Check sheet for the modelled part. Datum: model origin and axes. Units: mm. Face numbers are marked on the shaded views. A direction names the side the tool comes from. Coordinates: 2 decimals unless noted, no trailing zeros. Order: outer loops, then holes, each group sorted by start corner. A loop starts at its lowest first (then second) coordinate and runs counter-clockwise, first axis right, second up.
Autodesk Inventor part; units mm, degrees
ref_plane "YZ Plane" through (0, 0, 0) normal (1, 0, 0) x (0, 1, 0)
ref_plane "XZ Plane" through (0, 0, 0) normal (0, 1, 0) x (-1, 0, 0)
ref_plane "XY Plane" through (0, 0, 0) normal (0, 0, 1) x (1, 0, 0)
sketch "Sketch1" plane through (0, 0, 0) normal (0, 0, 1) x (1, 0, 0)
  line L0 (6.8523, -0.0001) -> (16.3773, -0.0001)
  line L1 (83.0523, -0.0001) -> (83.0523, 63.4999)
  line L2 (83.0523, 63.4999) -> (6.8523, 63.4999)
  line L3 (6.8523, 63.4999) -> (6.8523, -0.0001)
  line L4 (44.9523, 0) -> (60.8273, 0) construction
  line L5 (44.9523, 0) -> (60.8273, 0) construction
  line L6 (73.5273, -0.0001) -> (73.6164, -12.6997)
  line L7 (73.6164, -12.6997) -> (60.9164, -12.7)
  line L8 (60.9164, -12.7) -> (60.8273, 0)
  line L9 (73.5273, -0.0001) -> (83.0523, -0.0001)
  line L10 (44.9523, 0) -> (44.9523, 63.4999) construction
  line L11 (44.9523, 0) -> (29.0773, 0) construction
  line L12 (44.9523, 0) -> (29.0773, 0) construction
  line L13 (16.3773, -0.0001) -> (16.2881, -12.6997)
  line L14 (16.2881, -12.6997) -> (28.9881, -12.7)
  line L15 (28.9881, -12.7) -> (29.0773, 0)
  line L16 (29.0773, 0) -> (60.8273, 0)
  dimension "d10" = 76.2
  dimension "d11" = 63.5
  dimension "d12" = 15.875
  dimension "d13" = 0
  dimension "d14" = 12.7
  dimension "d15" = 12.7
extrude "Extrusion1" add sketch "Sketch1" along normal blind 12.7
sketch "Sketch2" plane through (0, 0, 12.7) normal (0, 0, 1) x (1, 0, 0)
  line L0 (72.65, -0.26) -> (16.25, -0.26) construction
  line L1 (16.25, -0.26) -> (16.25, 56.14) construction
  line L2 (16.25, 56.14) -> (72.65, 56.14) construction
  line L3 (72.65, 56.14) -> (72.65, -0.26) construction
  line L4 (16.25, -0.26) -> (72.65, 56.14) construction
  line L5 (68.02, 4.37) -> (20.88, 4.37) construction
  line L6 (20.88, 4.37) -> (20.88, 51.51) construction
  line L7 (20.88, 51.51) -> (68.02, 51.51) construction
  line L8 (68.02, 51.51) -> (68.02, 4.37) construction
  line L9 (68.02, 4.37) -> (20.88, 51.51) construction
  line L10 (20.88, 4.37) -> (68.02, 51.51) construction
  circle A0 centre (20.8494, 4.3394) radius 2.5
  circle A1 centre (20.88, 51.51) radius 2.5
  circle A2 centre (68.02, 51.51) radius 2.5
  circle A3 centre (68.02, 4.37) radius 2.5
  line L11 (29.0773, 0) -> (60.8273, 0) construction
  line L12 (44.9523, 0) -> (44.9523, 27.94) construction
  line L13 (44.9523, 0) -> (72.8923, 0) construction
  point P0 (0, 0)
  point P1 (44.45, 27.94)
  dimension "d18" = 47.14
  dimension "d19" = 47.14
  dimension "d20" = 5
  dimension "d21" = 5
  dimension "d22" = 5
  dimension "d23" = 5
  dimension "d24" = 27.94
  dimension "d25" = 90
extrude "Extrusion2" cut sketch "Sketch2" against normal through all
sketch "Sketch3" plane through (0, 0, 12.7) normal (0, 0, 1) x (1, 0, 0)
  circle A0 centre (44.45, 27.94) radius 19.05
  line L0 (29.0773, 0) -> (60.8273, 0) construction
  line L1 (44.9523, 0) -> (44.9523, 27.94) construction
  point P0 (0, 0)
  dimension "d28" = 38.1
  dimension "d29" = 27.94
extrude "Extrusion3" cut sketch "Sketch3" against normal blind 1.6
sketch "Sketch4" plane through (44.45, 27.94, 11.1) normal (0, 0, 1) x (1, 0, 0)
  circle A0 centre (0, 0) radius 12.7
  point P0 (-44.45, -27.94)
  dimension "d32" = 25.4
extrude "Extrusion4" cut sketch "Sketch4" against normal through all
sketch "Sketch5" plane through (0, 0, 12.7) normal (0, 0, 1) x (1, 0, 0)
  line L0 (29.0773, 0) -> (60.8273, 0) construction
  line L1 (44.9523, 0) -> (44.9523, 63.4999) construction
  line L2 (83.0523, 63.4999) -> (6.8523, 63.4999) construction
  line L3 (44.9523, 63.4999) -> (44.9523, 69.8499) construction
  line L4 (44.9523, 63.4999) -> (51.3023, 63.4999) construction
  line L5 (38.6023, 76.1999) -> (51.3023, 76.1999)
  line L6 (51.3023, 76.1999) -> (51.3023, 63.4999)
  line L7 (51.3023, 63.4999) -> (38.6023, 63.4999)
  line L8 (38.6023, 63.4999) -> (38.6023, 76.1999)
  line L9 (38.6023, 76.1999) -> (51.3023, 63.4999) construction
  line L10 (51.3023, 76.1999) -> (38.6023, 63.4999) construction
  point P0 (0, 0)
  dimension "d35" = 6.35
  dimension "d36" = 90
  dimension "d37" = 12.7
  dimension "d38" = 12.7
extrude "Extrusion5" add sketch "Sketch5" against normal blind 12.7
properties part number "Motor Bracket" material "PVC-Piping"
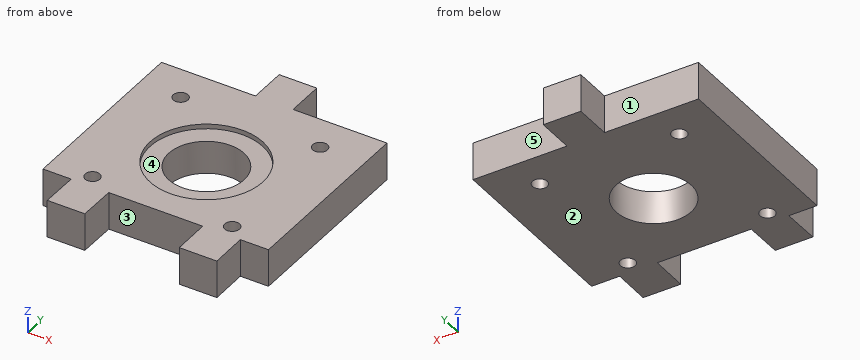
(1) Tool access check on the marked faces 1 and 2. Record the directions out of +Z, -Z, +X, -X, +Y, -Y that give a thin tool (end or side, any length) a straight path to the whole face; none if there is none.
Filled in:
face 1: +Z, -Z, -X, +Y
face 2: -Z, +X, -X, +Y, -Y
(2) Cross-section at B-B (x = 44.45). Enter the section's corners in (y, z), and give its area (3 significant figures).
Filled in:
outline: (0, 0) - (15.24, 0) - (15.24, 11.1) - (8.89, 11.1) - (8.89, 12.7) - (0, 12.7) - close; (40.64, 0) - (76.2, 0) - (76.2, 12.7) - (46.99, 12.7) - (46.99, 11.1) - (40.64, 11.1) - close
area: 625 mm2
(3) Release check for a two-part mould opening along Y. For the marked faces 3, 4 and 5 record: +Y half, -Y half, draft (parallel to the pull), parting line (faces both ways), or undercut.
Filled in:
face 3: -Y half
face 4: undercut
face 5: +Y half
(4) Cross-section at C-C (y = 27.94). Enter the section's corners in (x, z).
Filled in:
outline: (6.85, 0) - (31.75, 0) - (31.75, 11.1) - (25.4, 11.1) - (25.4, 12.7) - (6.85, 12.7) - close; (57.15, 0) - (83.05, 0) - (83.05, 12.7) - (63.5, 12.7) - (63.5, 11.1) - (57.15, 11.1) - close
(5) Cross-section at D-D (z = 3.25). Enter the section's corners in (x, y).
Filled in:
outline: (6.85, 0) - (16.38, 0) - (16.29, -12.7) - (28.99, -12.7) - (29.08, 0) - (60.83, 0) - (60.92, -12.7) - (73.62, -12.7) - (73.53, 0) - (83.05, 0) - (83.05, 63.5) - (51.3, 63.5) - (51.3, 76.2) - (38.6, 76.2) - (38.6, 63.5) - (6.85, 63.5) - close; hole circle Ø5 at (20.85, 4.34); hole circle Ø5 at (20.88, 51.51); hole circle Ø25.4 at (44.45, 27.94); hole circle Ø5 at (68.02, 4.37); hole circle Ø5 at (68.02, 51.51)
(6) Cross-section at A-A (y = 51.51). Enter the section's corners in (x, z).
Filled in:
outline: (6.85, 0) - (18.38, 0) - (18.38, 12.7) - (6.85, 12.7) - close; (23.38, 0) - (65.52, 0) - (65.52, 12.7) - (23.38, 12.7) - close; (70.52, 0) - (83.05, 0) - (83.05, 12.7) - (70.52, 12.7) - close
(7) Thickness scan on probe 1 along Y at (x, z) = (20.88, 3.5); probe 2 along Y at (x, z) = (68.02, 3.5); probe 3 along Y at (x, z) = (44.45, 8.5). Record the ranges inside material, lowest first.
Filled in:
probe 1: y = -12.7 to 1.84, 6.84 to 49.01, 54.01 to 63.5
probe 2: y = -12.7 to 1.87, 6.87 to 49.01, 54.01 to 63.5
probe 3: y = 0 to 15.24, 40.64 to 76.2
(8) Go/stop test with flat-tipped pins: P1, Ø20.5, axis at x = 44.45, y = 27.94, coming from the -Z side; P2, Ø5, axis at x = 22, z = 1.5, coming from the +Y side; P3, Ø1, axis at x = 53, z = 4.5, coming from the -Y side; P4, Ø6.5, axis at y = 72.5, z = 8.5, coming from the +X side. Record where each tip stops, or that it passes through.
Filled in:
P1: passes through
P2: stops at y = 63.5
P3: stops at y = 0
P4: stops at x = 51.3
